Read the model definition and answer for the solid it produces. Units are mm, in the model's axes. A direction names the side the tool comes from. Coordinates: 2 decimals unless noted, no trailing zeros. Write each loop counter-clockwise with the first axis right and the second up, starting at its lowest first coordinate (ties: lowest second). Pieces come first, ordered by that corner, then holes.
1) Find the intervals of material crossed by line 1 (Y direction, x = 13.5, z = 34.5); line 2 (Y direction, x = 22, z = 1.9); line 3 (Z direction, x = 6.5, y = -14), in increasing order.
2) Which of the six approach directions +Z, -Z, +X, -X, +Y, -Y give full straight-line access (tool end or side, diameter ignored) to faces 1 (the face through (20, 60, 5)), 2 (the face through (10, -59, 35)), 3 (the face through (0, 69, 30))?
3) The part is cut by section D-D (y = 26.5). Determine the outline of the cut face in (x, z).
4) Each of these flat-tipped pins is pushed along its axis until it touches: pin 1 Ø9.5 at (x, y) = (22, 58) entering from +Z; pin 2 Ø1.5 at (x, z) = (-1, 30.5) entering from -Y; pin 3 Ø13 at (y, z) = (66.5, 42.5) entering from -X. Where does it stop, or does it pass through?
5) Determine the mould class of faces 4 (the face through (21, -70, 35)), 5 (the face through (18.79, 74.93, 24.38)), 6 (the face through (-47.986, 1.148, 34.62)), 7 (the face through (0.9, -79.14, 29.55)) for opening direction X: +X half, -X half, draft (parallel to the pull), parting line (faces both ways), or undercut.
6) The part is cut by section C-C (x = -39.5). Determine the outline of the cut face in (y, z).
7) The part is cut by section A-A (y = 5). Determine the outline of the cut face in (x, z) (3 decimals), then the cut area to 3 significant figures.
8) The part is cut by section B-B (z = 55). Determine the outline of the cut face in (x, y), then the cut area to 3 significant figures.
from build123d import *

# Parameters (mm, degrees)
BOSS_EXTRUDE2_DEPTH     = 10
SKETCH3_R               = 2.25
CUT_EXTRUDE2_DEPTH      = 100.317672143
SKETCH4_R               = 3.6
CUT_EXTRUDE3_DEPTH      = 5
BOSS_EXTRUDE4_DEPTH     = 49.94
CUT_EXTRUDE5_DEPTH      = 172.629844724
CUT_EXTRUDE5_DEPTH_BACK = 172.629844724
SKETCH7_R               = 2.25
CUT_EXTRUDE6_DEPTH      = 111.715868781
CUT_EXTRUDE6_DEPTH_BACK = 111.715868781
SKETCH8_R               = 2.25
FILLET1_R               = 3
CUT_EXTRUDE7_DEPTH      = 116.571638389
CUT_EXTRUDE7_DEPTH_BACK = 5
SKETCH9_R               = 3.6


with BuildPart() as part:
    # Sketch1 → Boss-Extrude2 (new body)
    with BuildSketch(Plane(origin=(0, 0, 0), x_dir=(0, 1, 0), z_dir=(0, 0, 1))):
        with BuildLine():
            Line((-58, 0), (-80, 0))
            Line((-80, 0), (-80, -30))
            Line((-80, -30), (80, -30))
            Line((80, -30), (80, 0))
            Line((80, 0), (58, 0))
            ThreePointArc((58, 0), (0, 58), (-58, 0))
        make_face()
    extrude(amount=BOSS_EXTRUDE2_DEPTH)

    # Sketch3 → Cut-Extrude2 (cut, through all)
    with BuildSketch(Plane.XY.offset(10)):
        with Locations((13.625, -5)):
            Circle(SKETCH3_R)
        with Locations((-34.325, -5)):
            Circle(SKETCH3_R)
        with Locations(Location((-34.325, 5, 0), (0, 0, 180))):
            Circle(SKETCH3_R)
        with Locations(Location((13.625, 5, 0), (0, 0, 180))):
            Circle(SKETCH3_R)
    extrude(amount=-CUT_EXTRUDE2_DEPTH, mode=Mode.SUBTRACT)

    # Sketch4 → Cut-Extrude3 (cut)
    with BuildSketch(Plane(origin=(0, 0, 0), x_dir=(1, 0, 0), z_dir=(0, 0, -1))):
        with Locations(Location((-34.325, -5, 0), (0, 0, 180))):
            Circle(SKETCH4_R)
        with Locations(Location((-34.325, 5, 0), (0, 0, 180))):
            Circle(SKETCH4_R)
        with Locations(Location((13.625, 5, 0), (0, 0, 180))):
            Circle(SKETCH4_R)
        with Locations(Location((13.625, -5, 0), (0, 0, 180))):
            Circle(SKETCH4_R)
    extrude(amount=-CUT_EXTRUDE3_DEPTH, mode=Mode.SUBTRACT)

    # Sketch5 → Boss-Extrude4 (add)
    with BuildSketch(Plane.XY.offset(10)):
        with BuildLine():
            Line((10, -46.946778377), (10, -70))
            Line((10, -70), (20, -70))
            Line((20, -70), (30, -70))
            Line((30, -70), (30, -80))
            Line((30, -80), (0, -80))
            Line((0, -80), (0, -58))
            ThreePointArc((0, -58), (-58, 0), (0, 58))
            Line((0, 58), (0, 80))
            Line((0, 80), (30, 80))
            Line((30, 80), (30, 70))
            Line((30, 70), (20, 70))
            Line((20, 70), (10, 70))
            Line((10, 70), (10, 46.946778377))
            ThreePointArc((10, 46.946778377), (-48, 0), (10, -46.946778377))
        make_face()
    extrude(amount=BOSS_EXTRUDE4_DEPTH)

    # Sketch7 → Cut-Extrude5 (cut, two sides: drawn at the far end of the back side and taken through both)
    with BuildSketch(Plane(origin=(0, -70, 0), x_dir=(-1, 0, 0), z_dir=(0, 1, 0)).offset(-CUT_EXTRUDE5_DEPTH_BACK)):
        with Locations(Location((-20, 47.455, 0), (0, 0, 90))):
            Circle(SKETCH7_R)
        with Locations((-20, 22.485)):
            Circle(SKETCH7_R)
    extrude(amount=CUT_EXTRUDE5_DEPTH + CUT_EXTRUDE5_DEPTH_BACK, mode=Mode.SUBTRACT)

    # Sketch8 → Cut-Extrude6 (cut, two sides: drawn at the far end of the back side and taken through both)
    with BuildSketch(Plane.XY.offset(10).offset(-CUT_EXTRUDE6_DEPTH_BACK)):
        with Locations((22, -58)):
            Circle(SKETCH8_R)
        with Locations((22, 58)):
            Circle(SKETCH8_R)
    extrude(amount=CUT_EXTRUDE6_DEPTH + CUT_EXTRUDE6_DEPTH_BACK, mode=Mode.SUBTRACT)

    # Fillet1
    fillet1_edges = [part.edges().sort_by_distance(p)[0] for p in [
        (0, 80, 29.97),
        (0, -80, 29.97),
        (0, -58, 29.97),
        (0, 58, 29.97),
        (10, -70, 34.97),
        (10, -46.946778377, 34.97),
        (10, 46.946778377, 34.97),
        (10, 70, 34.97),
    ]]
    fillet(fillet1_edges, radius=FILLET1_R)

    # Sketch9 → Cut-Extrude7 (cut, two sides: drawn at the far end of the back side and taken through both)
    with BuildSketch(Plane(origin=(0, 0, 0), x_dir=(1, 0, 0), z_dir=(0, 0, -1)).offset(-CUT_EXTRUDE7_DEPTH_BACK)):
        with Locations((22, 58)):
            Circle(SKETCH9_R)
        with Locations((22, -58)):
            Circle(SKETCH9_R)
    extrude(amount=CUT_EXTRUDE7_DEPTH + CUT_EXTRUDE7_DEPTH_BACK, mode=Mode.SUBTRACT)


solid = part.part
Reported:
1. line 1: y = -80 to -70, 70 to 80
1. line 2: y = -80 to -61.6, -54.4 to 54.4, 61.6 to 80
1. line 3: z = 0 to 10
2. face 1: -Z
2. face 2: +Z, +X
2. face 3: +Z, -Z, -X, +Y
3. outline: (-51.59, 0) - (30, 0) - (30, 10) - (-40.02, 10) - (-40.02, 59.94) - (-51.59, 59.94) - close
4. pin 1: stops at z = 10
4. pin 2: stops at y = -59.73
4. pin 3: stops at x = -0.15
5. face 4: draft
5. face 5: undercut
5. face 6: undercut
5. face 7: -X half
6. outline: (-42.47, 0) - (42.47, 0) - (42.47, 59.94) - (27.27, 59.94) - (27.27, 10) - (-27.27, 10) - (-27.27, 59.94) - (-42.47, 59.94) - close
7. outline: (-57.784, 0) - (-37.925, 0) - (-37.925, 5) - (-36.575, 5) - (-36.575, 10) - (-47.739, 10) - (-47.739, 59.94) - (-57.784, 59.94) - close; (-32.075, 5) - (-30.725, 5) - (-30.725, 0) - (10.025, 0) - (10.025, 5) - (11.375, 5) - (11.375, 10) - (-32.075, 10) - close; (15.875, 5) - (17.225, 5) - (17.225, 0) - (30, 0) - (30, 10) - (15.875, 10) - close
7. area: 1,260 mm2
8. outline: (-2.85, -57.93) arc R3 cw to (0, -60.93) - (0, -77) arc R3 ccw to (3, -80) - (30, -80) - (30, -70) - (13, -70) arc R3 cw to (10, -67) - (10, -50.52) arc R3 ccw to (6.59, -47.55) arc R48 cw (long way) to (6.59, 47.55) arc R3 ccw to (10, 50.52) - (10, 67) arc R3 cw to (13, 70) - (30, 70) - (30, 80) - (3, 80) arc R3 ccw to (0, 77) - (0, 60.93) arc R3 cw to (-2.85, 57.93) arc R58 ccw to start
8. area: 2,710 mm2
